from build123d import *

# Parameters (mm, degrees)
SKETCH1_W           = 20
SKETCH1_H           = 20
BOSS_EXTRUDE1_DEPTH = 3
BOSS_EXTRUDE2_DEPTH = 17
SKETCH3_R           = 1.5
CUT_EXTRUDE1_DEPTH  = 17
SKETCH4_R           = 1.5
CUT_EXTRUDE2_DEPTH  = 17
SKETCH5_R           = 1.5
CUT_EXTRUDE3_DEPTH  = 17
FILLET1_R           = 7


with BuildPart() as part:
    # Sketch1 → Boss-Extrude1 (new body)
    with BuildSketch(Plane.XY):
        with Locations((10, 10)):
            Rectangle(SKETCH1_W, SKETCH1_H)
    extrude(amount=BOSS_EXTRUDE1_DEPTH)

    # Sketch2 → Boss-Extrude2 (add)
    with BuildSketch(Plane.XY.offset(3)):
        Polygon((0, 20), (3, 20), (3, 3), (20, 3), (20, 0), (0, 0), align=None)
    extrude(amount=BOSS_EXTRUDE2_DEPTH)

    # Sketch3 → Cut-Extrude1 (cut)
    with BuildSketch(Plane.ZY):
        with Locations((15, 15)):
            Circle(SKETCH3_R)
    extrude(amount=-CUT_EXTRUDE1_DEPTH, mode=Mode.SUBTRACT)

    # Sketch4 → Cut-Extrude2 (cut)
    with BuildSketch(Plane(origin=(0, 0, 0), x_dir=(-1, 0, 0), z_dir=(0, 0, -1))):
        with Locations((-15, 15)):
            Circle(SKETCH4_R)
    extrude(amount=-CUT_EXTRUDE2_DEPTH, mode=Mode.SUBTRACT)

    # Sketch5 → Cut-Extrude3 (cut)
    with BuildSketch(Plane(origin=(0, 0, 0), x_dir=(-1, 0, 0), z_dir=(0, -1, 0))):
        with Locations(Location((-15, -15, 0), (0, 0, 90))):
            Circle(SKETCH5_R)
    extrude(amount=-CUT_EXTRUDE3_DEPTH, mode=Mode.SUBTRACT)

    # Fillet1
    fillet1_edges = [part.edges().sort_by_distance(p)[0] for p in [
        (20, 1.5, 20),
        (1.5, 20, 20),
        (20, 20, 1.5),
    ]]
    fillet(fillet1_edges, radius=FILLET1_R)


solid = part.part
Design review of the part built by this model. Coordinates are the model's own, in mm. A direction names the side the tool comes from. Round coordinates to 2 decimals unless told otherwise and drop trailing zeros. Order: outer loops, then holes, each group sorted by start corner. A loop starts at its lowest first (then second) coordinate and runs counter-clockwise, first axis right, second up.
1) Consider section A-A (z = 15). State the section outline as (x, y) points.
The answers:
outline: (0, 0) - (13.5, 0) - (13.5, 3) - (3, 3) - (3, 13.5) - (0, 13.5) - close; (0, 16.5) - (3, 16.5) - (3, 19.71) - (0, 19.71) - close; (16.5, 0) - (19.71, 0) - (19.71, 3) - (16.5, 3) - close
2) Consider section C-C (y = 3.5). State the section outline as (x, z) points.
The answers:
outline: (0, 0) - (20, 0) - (20, 3) - (3, 3) - (3, 20) - (0, 20) - close
3) Clearance check with flat-ended pins moving along their axes: pin 1 Ø4 at (y, z) = (12.5, 8.5) entering from +X; pin 2 Ø1 at (x, y) = (14.5, 13) entering from +Z; pin 3 Ø5 at (x, z) = (8, 14.5) entering from +Y. State where each tip first meets the part, or that it passes through.
The answers:
pin 1: stops at x = 3
pin 2: stops at z = 3
pin 3: stops at y = 3
4) For L1, parallel to X at y = 5.75, z = 7.75; L2, parallel to Y at x = 0.95, z = 15, list the stretches that pass through material, from the lowest coordinate up.
The answers:
L1: x = 0 to 3
L2: y = 0 to 13.5, 16.5 to 19.71
5) Consider section B-B (x = 16). State the section outline as (y, z) points.
The answers:
outline: (0, 0) - (13.88, 0) - (13.88, 3) - (3, 3) - (3, 13.88) - (0, 13.88) - close; (0, 16.12) - (3, 16.12) - (3, 19.32) - (0, 19.32) - close; (16.12, 0) - (19.32, 0) - (19.32, 3) - (16.12, 3) - close
6) Draft analysis for pull direction Y (two halves, no side actions). For faces 1 (the cylindrical face through (15.07, 1.48, 16.5)), 2 (the cylindrical face through (1.48, 15.07, 13.5)), 3 (the flat face through (4, 20, 2)), state which applies: released by +Y, released by -Y, zero draft, split by the parting line, or undercut.
The answers:
face 1: zero draft
face 2: undercut
face 3: released by +Y
7) Machinability: for faces 4 (the flat face through (11, 12, 3)), 5 (the cylindrical face through (1.5, 18, 17.9)), which of the approach directions +Z, -Z, +X, -X, +Y, -Y give a long, thin tool a straight path to every point of the face, cutting with its end or side? Answer none if there is none.
The answers:
face 4: +Z, +X, +Y
face 5: +Z, +X, -X, +Y
